```python
from build123d import *

# Parameters (mm, degrees)
F1_DEPTH = 10
F2_R     = 0.25


with BuildPart() as f1:
    # F0 (on Top) → F1 (new body)
    with BuildSketch(Plane.XY):
        Polygon((27.5, 5), (-27.5, 5), (-27.5, -5), (-0.828427, -5), (0, -3), (0.828427, -5), (27.5, -5), align=None)
    extrude(amount=F1_DEPTH)

    # F2
    f2_edges = [f1.edges().sort_by_distance(p)[0] for p in [
        (0, -3, 5),
    ]]
    fillet(f2_edges, radius=F2_R)


solid = f1.part
```
Work out the finished part from the listing and answer in its coordinate system (mm). A direction names the side the tool comes from. Give positions to 0.01 mm unless a question says otherwise; leave off trailing zeros.
(1) Which of the six approach directions +Z, -Z, +X, -X, +Y, -Y give full straight-line access (tool end or side, diameter ignored) to faces 4 (the flat face through (0.526, -4.269, 4.93)), 5 (the flat face through (-14, -5, 5))?
Final values:
face 4: +Z, -Z, -Y
face 5: +Z, -Z, +X, -X, -Y
(2) The mould has two halves that part along X. Classify faces 1 (the flat face through (27.5, 0, 5)), 2 (the flat face through (0, 5, 5)), 3 (the flat face through (-0.534, -4.289, 4.93)): pulls with the +X half, pulls with the -X half, needs draft (parallel to the pull), parting line crosses it, or undercut.
Final values:
face 1: pulls with the +X half
face 2: needs draft
face 3: undercut
(3) Straight lines are drawn through the part: line 1 (X direction, y = -3.5, z = 3.5); line 2 (X direction, y = -4, z = 8.5). For each, find the intervals that lie inside material, in ascending order.
Final values:
line 1: x = -27.5 to -0.2, 0.2 to 27.5
line 2: x = -27.5 to -0.41, 0.41 to 27.5
